Check sheet for the modelled part. Datum: model origin and axes. Units: mm. A direction names the side the tool comes from. Round coordinates to 2 decimals unless told otherwise and drop trailing zeros. Loops run counter-clockwise (first coordinate to the right, second up) from the corner with the lowest first, then second, coordinate; pieces in that order, holes last. Notation, with made-up numbers: M 3.5,61.5 L 44.5,61.5 A19 ccw 44.5,85.5 Z; hole C 11,77.25 d1. An arc over 180 degrees is marked long. Write item = value, one per line. Start each with the question number.
(1) Go/stop test with flat-tipped pins: P1, Ø2, axis at x = 2.5, z = 27.5, coming from the +Y side; P2, Ø0.7, axis at y = 5.5, z = 27, coming from the -X side; P3, Ø0.5, axis at y = 6, z = 27, coming from the +X side. Record where each tip stops, or that it passes through.
(2) Cross-section at A-A on z = -21. Record the boundary of the cut face in (x, y) (3 decimals), plus the area to 3 significant figures.
(3) Scan lines: L1, parallel to Z at x = -12.5, y = 1.25 (3 decimals); L2, parallel to X at y = 1.75, z = -18.5 (3 decimals); L3, parallel to Z at x = -13.5, y = 6. Record each from-to range of solid material in increasing order. Write a range as from..to.
(4) Mould release check, pull along Z, two halves, no side actions. Record for faces 1 (the face through (45, 3, 0)), 2 (the face through (-1, 3, 30)), 3 (the face through (-1, 2, -26.825)): pulls with the +Z half, pulls with the -Z half, needs draft (parallel to the pull), parting line crosses it, or undercut.
(5) Cross-section at B-B on y = 1. Record the boundary of the cut face in (x, z) (3 decimals), plus the area to 3 significant figures.
(6) Set-up check for faces 4 (the face through (-43.809, 3.131, 28.745)), 5 (the face through (0, 4.762, -28)), 6 (the face through (41.825, 3, 0)): record each of +Z, -Z, +X, -X, +Y, -Y from which the full face is reachable in a straight line by a thin tool's end or side.
from build123d import *

# Parameters (mm, degrees)
BOSS_EXTRUDE3_DEPTH = 6.35
SKETCH5_R           = 1.4224
SKETCH5_R_2         = 1.4732
CUT_EXTRUDE2_DEPTH  = 55.454774814
CUT_EXTRUDE3_DEPTH  = 1.5875


with BuildPart() as part:
    # Sketch2 → Boss-Extrude3 (new body)
    with BuildSketch(Plane(origin=(0, 0, 0), x_dir=(1, 0, 0), z_dir=(0, 1, 0))):
        with BuildLine():
            Line((-45, 25.825), (-45, -25.825))
            ThreePointArc((-45, -25.825), (-43.777170811, -28.777170811), (-40.825, -30))
            Line((-40.825, -30), (40.825, -30))
            ThreePointArc((40.825, -30), (43.777170811, -28.777170811), (45, -25.825))
            Line((45, -25.825), (45, 25.825))
            ThreePointArc((45, 25.825), (43.777170811, 28.777170811), (40.825, 30))
            Line((40.825, 30), (-40.825, 30))
            ThreePointArc((-40.825, 30), (-43.777170811, 28.777170811), (-45, 25.825))
        make_face()
        with BuildLine():
            Line((-41.825, -25.825), (-41.825, 25.825))
            ThreePointArc((-41.825, 25.825), (-41.532106781, 26.532106781), (-40.825, 26.825))
            Line((-40.825, 26.825), (40.825, 26.825))
            ThreePointArc((40.825, 26.825), (41.532106781, 26.532106781), (41.825, 25.825))
            Line((41.825, 25.825), (41.825, -25.825))
            ThreePointArc((41.825, -25.825), (41.532106781, -26.532106781), (40.825, -26.825))
            Line((40.825, -26.825), (-40.825, -26.825))
            ThreePointArc((-40.825, -26.825), (-41.532106781, -26.532106781), (-41.825, -25.825))
        make_face(mode=Mode.SUBTRACT)
    extrude(amount=BOSS_EXTRUDE3_DEPTH)

    # Sketch5 → Cut-Extrude2 (cut, through all)
    with BuildSketch(Plane.XZ):
        with Locations((-40.825, 25.825)):
            Circle(SKETCH5_R)
        with Locations((40.825, 25.81487963)):
            Circle(SKETCH5_R_2)
        with Locations((40.825, -25.825)):
            Circle(SKETCH5_R_2)
        with Locations((-40.825, -25.81356336)):
            Circle(SKETCH5_R_2)
    extrude(amount=-CUT_EXTRUDE2_DEPTH, mode=Mode.SUBTRACT)

    # Sketch7 → Cut-Extrude3 (cut)
    with BuildSketch(Plane(origin=(0, 6.35, 0), x_dir=(1, 0, 0), z_dir=(0, 1, 0))):
        with BuildLine():
            Line((-35.00387248, 27.407439815), (-35.00387248, 25.81487963))
            Line((-35.00387248, 25.81487963), (34.993187521, 25.81487963))
            Line((34.993187521, 25.81487963), (34.993187521, 27.407439815))
            ThreePointArc((34.993187521, 27.407439815), (34.627070997, 28.291323292), (33.743187521, 28.657439815))
            Line((33.743187521, 28.657439815), (-33.75387248, 28.657439815))
            ThreePointArc((-33.75387248, 28.657439815), (-34.637755957, 28.291323292), (-35.00387248, 27.407439815))
        make_face()
        with BuildLine():
            Line((-43.6625, -18.823576125), (-43.6625, 18.721630511))
            ThreePointArc((-43.6625, 18.721630511), (-43.296383476, 19.605513988), (-42.4125, 19.971630511))
            Line((-42.4125, 19.971630511), (-40.825, 19.971630511))
            Line((-40.825, 19.971630511), (-40.825, -20.073576125))
            Line((-40.825, -20.073576125), (-42.4125, -20.073576125))
            ThreePointArc((-42.4125, -20.073576125), (-43.296383476, -19.707459601), (-43.6625, -18.823576125))
        make_face()
        with BuildLine():
            Line((40.825, 14.983067151), (42.4125, 14.983067151))
            ThreePointArc((42.4125, 14.983067151), (43.296383476, 14.616950627), (43.6625, 13.733067151))
            Line((43.6625, 13.733067151), (43.6625, -13.743187521))
            ThreePointArc((43.6625, -13.743187521), (43.296383476, -14.627070997), (42.4125, -14.993187521))
            Line((42.4125, -14.993187521), (40.825, -14.993187521))
            Line((40.825, -14.993187521), (40.825, 14.983067151))
        make_face()
        with BuildLine():
            Line((-28.813455755, -28.667560185), (28.75263109, -28.667560185))
            ThreePointArc((28.75263109, -28.667560185), (29.636514567, -28.301443661), (30.00263109, -27.417560185))
            Line((30.00263109, -27.417560185), (30.00263109, -25.83512037))
            Line((30.00263109, -25.83512037), (-30.063455755, -25.83512037))
            Line((-30.063455755, -25.83512037), (-30.063455755, -27.417560185))
            ThreePointArc((-30.063455755, -27.417560185), (-29.697339231, -28.301443661), (-28.813455755, -28.667560185))
        make_face()
    extrude(amount=-CUT_EXTRUDE3_DEPTH, mode=Mode.SUBTRACT)


solid = part.part
Result:
q1.P1 = 4.76
q1.P2 = -44.92
q1.P3 = 44.9
q2.outline = M -45,0 L -41.825,0 L -41.825,6.35 L -45,6.35 Z; M 41.825,0 L 45,0 L 45,6.35 L 41.825,6.35 Z
q2.area = 40.3 mm^2
q3.L1 = -30..-26.825, 26.825..30
q3.L2 = -45..-41.825, 41.825..45
q3.L3 = -30..-28.66, 28.67..30
q4.face_1 = needs draft
q4.face_2 = pulls with the +Z half
q4.face_3 = undercut
q5.outline = M -45,-25.825 A4.175 ccw -40.825,-30 L 40.825,-30 A4.175 ccw 45,-25.825 L 45,25.825 A4.175 ccw 40.825,30 L -40.825,30 A4.175 ccw -45,25.825 Z; hole M -41.825,-24.732 A1.473 ccw long -39.754,-26.825 L 39.743,-26.825 A1.473 ccw long 41.825,-24.743 L 41.825,24.733 A1.473 ccw long 39.753,26.825 L -39.813,26.825 A1.422 ccw long -41.825,24.813 Z
q5.area = 892 mm^2
q6.face_4 = +Z, -X, +Y, -Y
q6.face_5 = +Y
q6.face_6 = +Y, -Y
